Answer from the drawing. Dimensions are ordinates in mm from the lowest x, y and z of the part. A direction names the side the tool comes from. Coordinates: 2 decimals unless noted, no trailing zeros. Write each loop counter-clockwise with the first axis right and the second up, starting at its lowest first coordinate (ties: lowest second). Pieces come first, ordered by that corner, then holes.
(1) The part is cut by section C-C, the plane y = 26. Determine the outline of the cut face in (x, z).
(2) The part is cut by section D-D, the plane x = 15. Determine the outline of the cut face in (y, z).
(3) The part is cut by section B-B, the plane x = 10. Determine the outline of the cut face in (y, z), and give its area (3 significant figures).
(4) The part is cut by section A-A, the plane z = 13. Determine the outline of the cut face in (x, y).
(5) Determine the mould class of the marked faces 3, 4 and 5 for opening direction Y: pulls with the +Y half, pulls with the -Y half, needs draft (parallel to the pull), parting line crosses it, or undercut.
(6) Given pin 1 (8 mm diameter, centred on x = 11.5, y = 28, fed in from -Z); pin 2 (3 mm diameter, centred on x = 4.5, y = 11, fed in from +Z); pin 3 (10 mm diameter, centred on x = 9, z = 12, fed in from +Y), each flat-ended and moving along its own axis, determine where each tip first touches the part or whether it passes through.
(7) Which of the six approach directions +Z, -Z, +X, -X, +Y, -Y give full straight-line access (tool end or side, diameter ignored) to the marked faces 1 and 2?
(8) Straight lines are drawn through the part: line 1 along X through (y, z) = (1.9, 13); line 2 along Y through (x, z) = (10, 0.85); line 3 along Z through (x, y) = (18, 13.5). For each, find the intervals that lie inside material, in ascending order.
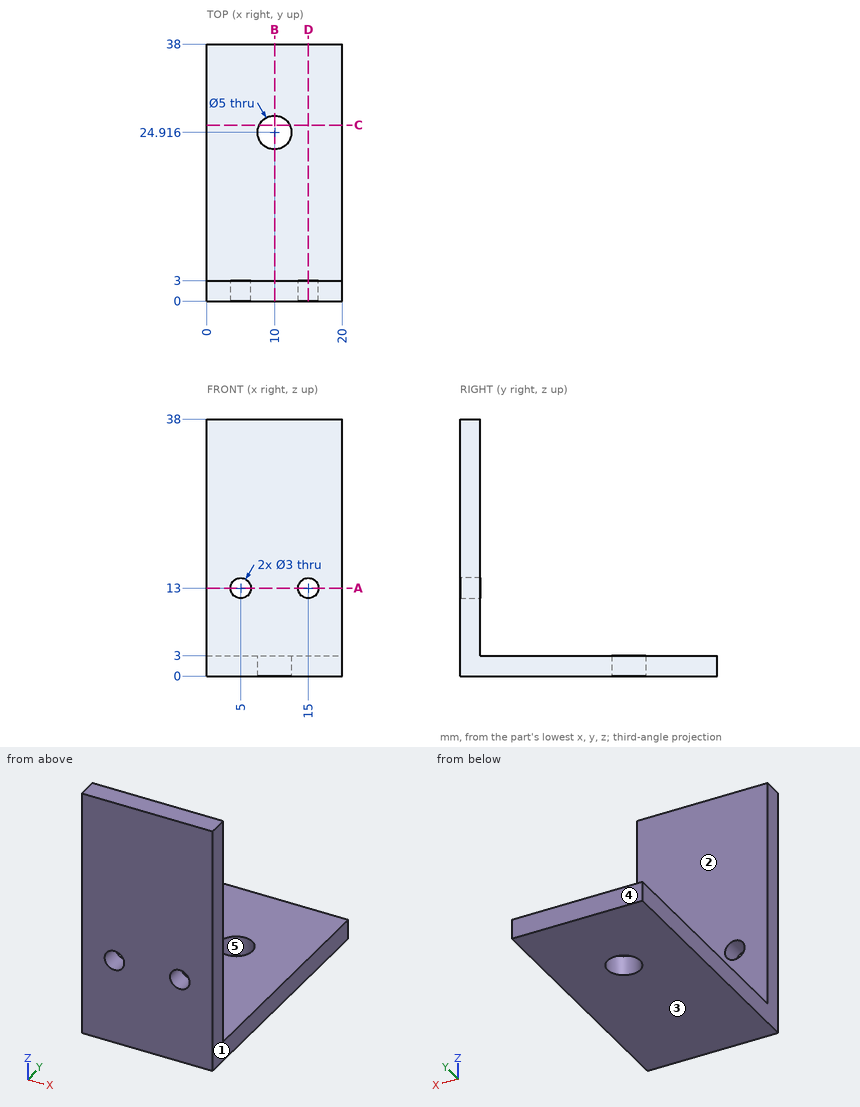
Computed:
1. outline: (0, 0) - (7.75, 0) - (7.75, 3) - (0, 3) - close; (12.25, 0) - (20, 0) - (20, 3) - (12.25, 3) - close
2. outline: (0, 0) - (38, 0) - (38, 3) - (3, 3) - (3, 11.5) - (0, 11.5) - close; (0, 14.5) - (3, 14.5) - (3, 38) - (0, 38) - close
3. outline: (0, 0) - (22.42, 0) - (22.42, 3) - (3, 3) - (3, 38) - (0, 38) - close; (27.42, 0) - (38, 0) - (38, 3) - (27.42, 3) - close
3. area: 204 mm2
4. outline: (0, 0) - (3.5, 0) - (3.5, 3) - (0, 3) - close; (6.5, 0) - (13.5, 0) - (13.5, 3) - (6.5, 3) - close; (16.5, 0) - (20, 0) - (20, 3) - (16.5, 3) - close
5. face 3: needs draft
5. face 4: pulls with the +Y half
5. face 5: undercut
6. pin 1: stops at z = 0
6. pin 2: stops at z = 3
6. pin 3: stops at y = 3
7. face 1: +Z, -Z, +X, +Y, -Y
7. face 2: +Z, +X, -X, +Y
8. line 1: x = 0 to 3.5, 6.5 to 13.5, 16.5 to 20
8. line 2: y = 0 to 22.42, 27.42 to 38
8. line 3: z = 0 to 3
